from build123d import *

# Parameters (mm, degrees)
F0_R     = 144
F0_R_2   = 10.1
F0_R_3   = 27.5
F0_R_4   = 6
F3_DEPTH = 25


with BuildPart() as f2:
    # F1 (on Right) → F2 (revolve)
    with BuildSketch(Plane.YZ):
        Polygon((-22, 0), (0, 0), (0, 144), (-11, 144), (-11, 95.5), (-22, 77.5), align=None)
    revolve(axis=Axis((0, -11, 0), (0, 1, 0)))

    # F0 (on Front) → F3 (intersect)
    with BuildSketch(Plane.XZ):
        Circle(F0_R)
        with Locations((-69.282032, -40)):
            Circle(F0_R_2, mode=Mode.SUBTRACT)
        with BuildLine():
            ThreePointArc((-35.355339, -28.991378), (-35.344887, -21.202779), (-27.556343, -21.234136))
            Line((-27.556343, -21.234136), (-21.738307, -27.114974))
            ThreePointArc((-21.738307, -27.114974), (-21.192382, -27.598098), (-20.715148, -28.149178))
            ThreePointArc((-20.715148, -28.149178), (-19.887922, -29.716864), (-19.602291, -31.466252))
            ThreePointArc((-19.602291, -31.466252), (-22.998539, -36.548006), (-28.99292, -35.353796))
            Line((-28.99292, -35.353796), (-35.355339, -28.991378))
        make_face(mode=Mode.SUBTRACT)
        with Locations((0, -80)):
            Circle(F0_R_2, mode=Mode.SUBTRACT)
        with Locations((69.282032, -40)):
            Circle(F0_R_2, mode=Mode.SUBTRACT)
        with BuildLine():
            ThreePointArc((28.991378, -35.355339), (21.202779, -35.344887), (21.234136, -27.556343))
            Line((21.234136, -27.556343), (27.114974, -21.738307))
            ThreePointArc((27.114974, -21.738307), (27.598098, -21.192382), (28.149178, -20.715148))
            ThreePointArc((28.149178, -20.715148), (33.916363, -20.178171), (36.966252, -25.102291))
            ThreePointArc((36.966252, -25.102291), (36.547172, -27.208057), (35.353796, -28.99292))
            Line((35.353796, -28.99292), (28.991378, -35.355339))
        make_face(mode=Mode.SUBTRACT)
        with BuildLine():
            ThreePointArc((-28.991378, 35.355339), (-22.997532, 36.547589), (-19.602291, 31.466252))
            ThreePointArc((-19.602291, 31.466252), (-20.026621, 29.347862), (-21.234136, 27.556343))
            Line((-21.234136, 27.556343), (-27.114974, 21.738307))
            ThreePointArc((-27.114974, 21.738307), (-27.598098, 21.192382), (-28.149178, 20.715148))
            ThreePointArc((-28.149178, 20.715148), (-35.614955, 21.491437), (-35.353796, 28.99292))
            Line((-35.353796, 28.99292), (-28.991378, 35.355339))
        make_face(mode=Mode.SUBTRACT)
        with Locations((-69.282032, 40)):
            Circle(F0_R_2, mode=Mode.SUBTRACT)
        Circle(F0_R_3, mode=Mode.SUBTRACT)
        with BuildLine():
            ThreePointArc((35.355339, 28.991378), (36.547589, 27.20705), (36.966252, 25.102291))
            ThreePointArc((36.966252, 25.102291), (33.557364, 20.015322), (27.556343, 21.234136))
            Line((27.556343, 21.234136), (21.738307, 27.114974))
            ThreePointArc((21.738307, 27.114974), (21.192382, 27.598098), (20.715148, 28.149178))
            ThreePointArc((20.715148, 28.149178), (21.491437, 35.614955), (28.99292, 35.353796))
            Line((28.99292, 35.353796), (35.355339, 28.991378))
        make_face(mode=Mode.SUBTRACT)
        with Locations((0, 40)):
            Circle(F0_R_4, mode=Mode.SUBTRACT)
        with Locations((69.282032, 40)):
            Circle(F0_R_2, mode=Mode.SUBTRACT)
        with Locations((0, 80)):
            Circle(F0_R_2, mode=Mode.SUBTRACT)
    extrude(amount=F3_DEPTH, mode=Mode.INTERSECT)


solid = f2.part
For this review, take the finished solid that the model builds, in its own axes (mm). A direction names the side the tool comes from. Give positions to 0.01 mm unless a question says otherwise; leave off trailing zeros. Loops run counter-clockwise (first coordinate to the right, second up) from the corner with the lowest first, then second, coordinate; pieces in that order, holes last.
Item 1: Take a section at B-B, the plane z = 0. State the section outline as (x, y) points.
Item 2: Take a section at C-C, the plane x = 118.5. State the section outline as (y, z) points.
Item 3: Take a section at A-A, the plane y = -7. Give the number of separate pieces and of enclosed holes in the cut face, and give its area (3 significant figures).
Item 4: Insertion check: pin 1 (10 mm diameter, centred on x = 97, y = -5, fed in from -Z); pin 2 (18 mm diameter, centred on x = 69.28, z = 40, fed in from +Y); pin 3 (1.5 mm diameter, centred on y = -11, z = -113, fed in from -X); pin 4 (8 mm diameter, centred on y = -11.5, z = 23, fed in from +X). Each pin has a flat end and moves straight along its axis. Give the tip position at first contact, or say it passes through.
Item 5: Take a section at D-D, the plane z = -119. State the section outline as (x, y) points.
Item 6: Tool access review of faces 4 (the flat face through (32.13, -10.846, 32.217)), 5 (the flat face through (2, 0, -30)): name each direction out of +Z, -Z, +X, -X, +Y, -Y from which nothing blocks a thin tool from reaching the whole face with its end or side.
Item 7: For line 1 along Z through (x, y) = (22.5, -12.75); line 2 along Z through (x, y) = (4, -18); line 3 along Z through (x, y) = (0, -14), list the stretches that pass through material, from the lowest coordinate up.
Item 8: Draft analysis for pull direction X (two halves, no side actions). For faces 1 (the cylindrical face through (142.775, -5.577, -18.746)), 2 (the cylindrical face through (-2.19, -10.85, 70.14)), 3 (the flat face through (-94, -11, 30)), state which applies: +X half, -X half, draft (parallel to the pull), parting line (faces both ways), or undercut.
Calculated:
1. outline: (-144, -11) - (-95.5, -11) - (-77.5, -22) - (-27.5, -22) - (-27.5, 0) - (-144, 0) - close; (27.5, -22) - (77.5, -22) - (95.5, -11) - (144, -11) - (144, 0) - (27.5, 0) - close
2. outline: (-11, -81.82) - (0, -81.82) - (0, 81.82) - (-11, 81.82) - close
3. separate pieces: 1
3. enclosed holes: 12
3. area: 60,000 mm2
4. pin 1: stops at z = -110.78
4. pin 2: passes through
4. pin 3: stops at x = -90.2
4. pin 4: stops at x = 142.74
5. outline: (-81.09, -11) - (81.09, -11) - (81.09, 0) - (-81.09, 0) - close
6. face 4: +Y, -Y
6. face 5: +Z, -Z, +X, -X, +Y
7. line 1: z = -89.86 to -36.31, -26.3 to -15.81, 15.81 to 26.35, 36.31 to 89.86
7. line 2: z = -70.73 to -27.21, 27.21 to 35.53, 44.47 to 70.73
7. line 3: z = -90.59 to -90.1, -69.9 to -27.5, 27.5 to 34, 46 to 69.9, 90.1 to 90.59
8. face 1: parting line
8. face 2: undercut
8. face 3: draft
